Answer from the drawing. Dimensions are ordinates in mm from the lowest x, y and z of the part. A direction names the side the tool comes from. Coordinates: 2 decimals unless noted, no trailing zeros. Loops run counter-clockwise (first coordinate to the right, second up) from the corner with the lowest first, then second, coordinate; pieces in that order, holes last. Notation, with made-up numbers: (24, 50) - (43, 50) arc R32 ccw to (43, 79) - close; hole circle Ø9 at (14.25, 1). An arc over 180 degrees is marked (long way). Use one line per item in the form item = value. Start each with the question number.
1) A cutting plane is placed at D-D (z = 35.2). Give the vertices of the cut face in (x, y), and give its area (3 significant figures).
2) Each of these flat-tipped pins is pushed along its axis until it touches: P1, Ø5, axis at y = 6.5, z = 31, coming from the -X side; P2, Ø1, axis at x = 4, z = 6.5, coming from the +Y side; P3, Ø4, axis at x = 5, z = 35.2, coming from the +Y side. Where does it stop, or does it pass through?
3) Which of the six approach directions +Z, -Z, +X, -X, +Y, -Y give full straight-line access (tool end or side, diameter ignored) to the marked faces 5, 6 and 7?
4) The mould has two halves that part along Z. Classify the marked faces 1, 2, 3 and 4: released by +Z, released by -Z, zero draft, split by the parting line, or undercut.
5) A cutting plane is placed at C-C (x = 2.5). Give the vertices of the cut face in (y, z), and give its area (3 significant figures).
6) A cutting plane is placed at B-B (y = 5). Give the vertices of the cut face in (x, z), and give its area (3 significant figures).
7) A cutting plane is placed at A-A (x = 4.25). Give the vertices of the cut face in (y, z).
8) Consider line 1 (Z direction, x = 5, y = 5.75); line 2 (X direction, y = 4.75, z = 35.2); line 3 (Z direction, x = 5.25, y = 1.5). Determine where each line is inside the solid, lowest interval first.
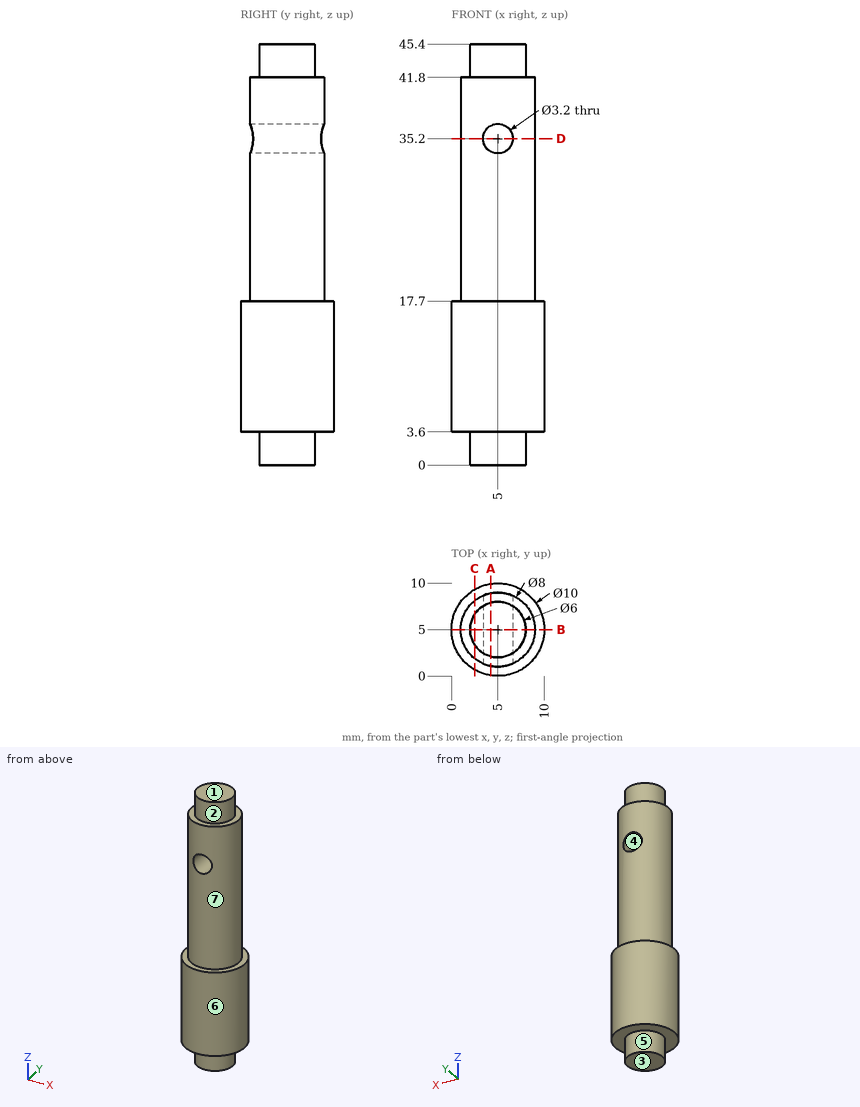
Found:
q1.outline = (3.4, 1.33) - (3.4, 8.67) arc R4 ccw to start; (6.6, 1.33) arc R4 ccw to (6.6, 8.67) - close
q1.area = 25.4 mm^2
q2.P1 = 1
q2.P2 = 9.97
q2.P3 = 9
q3.face_5 = -Z
q3.face_6 = +Z, -Z
q3.face_7 = +Z
q4.face_1 = released by +Z
q4.face_2 = zero draft
q4.face_3 = released by -Z
q4.face_4 = undercut
q5.outline = (0.67, 3.6) - (3.34, 3.6) - (3.34, 0) - (6.66, 0) - (6.66, 3.6) - (9.33, 3.6) - (9.33, 17.7) - (8.12, 17.7) - (8.12, 41.8) - (6.66, 41.8) - (6.66, 45.4) - (3.34, 45.4) - (3.34, 41.8) - (1.88, 41.8) - (1.88, 17.7) - (0.67, 17.7) - close
q5.area = 296 mm^2
q6.outline = (0, 3.6) - (2, 3.6) - (2, 0) - (8, 0) - (8, 3.6) - (10, 3.6) - (10, 17.7) - (9, 17.7) - (9, 41.8) - (8, 41.8) - (8, 45.4) - (2, 45.4) - (2, 41.8) - (1, 41.8) - (1, 17.7) - (0, 17.7) - close; hole circle Ø3.2 at (5, 35.2)
q6.area = 369 mm^2
q7.outline = (0.06, 3.6) - (2.1, 3.6) - (2.1, 0) - (7.9, 0) - (7.9, 3.6) - (9.94, 3.6) - (9.94, 17.7) - (8.93, 17.7) - (8.93, 33.79) - (1.07, 33.79) - (1.07, 17.7) - (0.06, 17.7) - close; (1.07, 36.61) - (8.93, 36.61) - (8.93, 41.8) - (7.9, 41.8) - (7.9, 45.4) - (2.1, 45.4) - (2.1, 41.8) - (1.07, 41.8) - close
q8.line_1 = 0 to 33.6, 36.8 to 45.4
q8.line_2 = 1.01 to 3.4, 6.6 to 8.99
q8.line_3 = 3.6 to 33.62, 36.78 to 41.8
